Geometry: final body of the model. Coordinates: model frame, mm. Face numbers are marked on the shaded views. A direction names the side the tool comes from. Coordinates: 2 decimals unless noted, no trailing zeros. Order: outer loops, then holes, each group sorted by start corner. A loop starts at its lowest first (then second) coordinate and runs counter-clockwise, first axis right, second up. Notation, with made-up numbers: (60.5, 46) -> (94.5, 46) arc R16 cw to (94.5, 77) -> close; hole circle Ø4 at (52, 55.25). An arc over 180 degrees is marked (long way). Answer in a Markdown table with one row per item. Add a question column.
1) Ray query, line 1 (X direction, y = -0.75, z = -18); line 2 (X direction, y = -2, z = -5); line 3 (Z direction, x = 59, y = -7). Return the intervals inside material, ascending. Write a range as from..to.
2) Section query A-A on x = -10.5. Return the cut outline in (y, z) (3 decimals), then the cut area to 3 significant figures.
3) Section query B-B on x = -40.5. Return the cut outline in (y, z) (3 decimals), then the cut area to 3 significant figures.
4) Section query C-C on z = -12.5. Count the separate pieces of the cut face and the enclosed holes in it, then the cut area to 3 significant figures.
5) Contact query for flat-ended pins moving along their axis: P1, Ø8, axis at x = -64.17, y = -2.89, coming from the -Z side; P2, Ø0.7, axis at x = 122.5, z = -12, coming from the +Y side (3 decimals); P3, Ø1.5, axis at x = -33, z = -14, coming from the +Y side (3 decimals). Output: stop coordinate, or through.
6) Set-up query: the marked faces 1, 2 and 3. Return all of +Z, -Z, +X, -X, +Y, -Y with unobstructed straight access to the full face (end or side cutting, diameter ignored); none if empty.
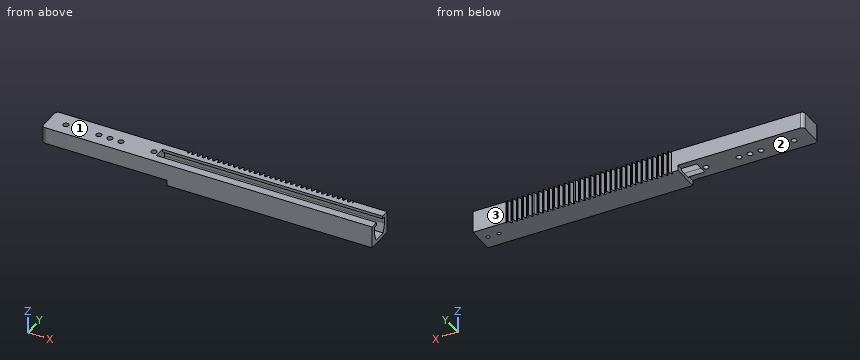
```python
from build123d import *

# Parameters (mm, degrees)
BLANKSKE_W              = 150
BLANKSKE_H              = 11.5
BLANK_DEPTH             = 20
TOOTHCUTSIM_DEPTH       = 152.763796737
TEETHCUTS_COUNT         = 33
TEETHCUTS_PITCH         = 4.712388975
BOSS_EXTRUDE1_DEPTH     = 20
BOSS_EXTRUDE2_DEPTH     = 20
SKETCH3_W               = 190
SKETCH3_H               = 20
BOSS_EXTRUDE3_DEPTH     = 14.285
CUT_EXTRUDE1_DEPTH      = 192.583040024
SKETCH6_W               = 20
SKETCH6_H               = 24.61
BOSS_EXTRUDE4_DEPTH     = 140
BOSS_EXTRUDE5_DEPTH     = 10
SKETCH9_R               = 2.5
CUT_EXTRUDE2_DEPTH      = 182.670199056
CUT_EXTRUDE5_DEPTH      = 341.88716788
CUT_EXTRUDE5_DEPTH_BACK = 154
SKETCH15_W              = 2.5
SKETCH15_H              = 15
BOSS_EXTRUDE9_DEPTH     = 10
SKETCH16_R              = 2
CUT_EXTRUDE7_DEPTH      = 10
SKETCH17_W              = 15
SKETCH17_H              = 10
CUT_EXTRUDE8_DEPTH      = 177
SKETCH20_W              = 15
SKETCH20_H              = 24.61
CUT_EXTRUDE9_DEPTH      = 40
FILLET2_R               = 3
SKETCH21_R              = 1.6
CUT_EXTRUDE10_DEPTH     = 40


with BuildPart() as part:
    # BlankSke → Blank (new body)
    with BuildSketch(Plane.XY):
        with Locations((75, 5.75)):
            Rectangle(BLANKSKE_W, BLANKSKE_H)
    extrude(amount=-BLANK_DEPTH)

    # TooCutSkeSim → ToothCutSim (cut, through all)
    with BuildSketch(Plane.XY):
        Polygon((0.654653055, 8.125), (-0.654653055, 8.125), (-1.892297439, 11.5254), (1.892297439, 11.5254), align=None)
    toothcutsim = extrude(amount=-TOOTHCUTSIM_DEPTH, mode=Mode.SUBTRACT)

    # TeethCuts: ToothCutSim ×33
    with Locations(*[(i * TEETHCUTS_PITCH, 0, 0) for i in range(1, TEETHCUTS_COUNT)]):
        add(toothcutsim, mode=Mode.SUBTRACT)

    # Sketch1 → Boss-Extrude1 (add)
    with BuildSketch(Plane(origin=(150, 0, 0), x_dir=(0, 0, -1), z_dir=(1, 0, 0))):
        Polygon((0, 8.514576213), (0, 10.714576213), (20, 10.714576213), (20, 0), (0, 0), align=None)
    extrude(amount=BOSS_EXTRUDE1_DEPTH)

    # Sketch2 → Boss-Extrude2 (add)
    with BuildSketch(Plane.ZY):
        Polygon((-20, 8.125), (-20, 10.325), (0, 10.325), (0, 0), (-20, 0), align=None)
    extrude(amount=BOSS_EXTRUDE2_DEPTH)

    # Sketch3 → Boss-Extrude3 (add)
    with BuildSketch(Plane.XZ):
        with Locations((75, -10)):
            Rectangle(SKETCH3_W, SKETCH3_H)
    extrude(amount=BOSS_EXTRUDE3_DEPTH)

    # Sketch4 → Cut-Extrude1 (cut, through all)
    with BuildSketch(Plane(origin=(170, 0, 0), x_dir=(0, 0, -1), z_dir=(1, 0, 0))):
        Polygon((2.5, -6.785211894), (2.5, -10.385211894), (8.7, -10.385211894), (16.7, -7.785211894), (16.7, -1.785211894), (16.7, 4.214788106), (8.7, 6.814788106), (2.5, 6.814788106), (2.5, 3.214788106), (0, 3.214788106), (0, -1.785211894), (0, -6.785211894), align=None)
    extrude(amount=-CUT_EXTRUDE1_DEPTH, mode=Mode.SUBTRACT)

    # Sketch6 → Boss-Extrude4 (add)
    with BuildSketch(Plane.ZY.offset(20)):
        with Locations((-10, -1.98)):
            Rectangle(SKETCH6_W, SKETCH6_H)
    extrude(amount=BOSS_EXTRUDE4_DEPTH)

    # Sketch8 → Boss-Extrude5 (add)
    with BuildSketch(Plane(origin=(170, 0, 0), x_dir=(0, 0, -1), z_dir=(1, 0, 0))):
        Polygon((20, 10.714576213), (20, -14.285), (0, -14.285), (0, -6.785211894), (2.5, -6.785211894), (2.5, -10.385211894), (8.7, -10.385211894), (16.7, -7.785211894), (16.7, 4.214788106), (8.7, 6.814788106), (2.5, 6.814788106), (2.5, 3.214788106), (0, 3.214788106), (0, 10.714576213), align=None)
    extrude(amount=BOSS_EXTRUDE5_DEPTH)

    # Sketch9 → Cut-Extrude2 (cut, through all)
    with BuildSketch(Plane(origin=(0, 0, -20), x_dir=(-1, 0, 0), z_dir=(0, 0, -1))):
        with Locations((24.169323408, -2.889762756)):
            Circle(SKETCH9_R)
        with Locations((54.169323408, -2.889762756)):
            Circle(SKETCH9_R)
        with Locations((64.169323408, -2.889762756)):
            Circle(SKETCH9_R)
        with Locations((74.169323408, -2.889762756)):
            Circle(SKETCH9_R)
        with Locations((104.169323408, -2.889762756)):
            Circle(SKETCH9_R)
    extrude(amount=-CUT_EXTRUDE2_DEPTH, mode=Mode.SUBTRACT)

    # Sketch10 → Cut-Extrude5 (cut, two sides: drawn at the far end of the back side and taken through both)
    with BuildSketch(Plane.ZY.offset(160).offset(-CUT_EXTRUDE5_DEPTH_BACK)):
        Polygon((-20, -14.285), (-15, -14.285), (-15, 10.325), (-15, 11.5), (-20, 11.5), (-20, 10.325), align=None)
    extrude(amount=CUT_EXTRUDE5_DEPTH + CUT_EXTRUDE5_DEPTH_BACK, mode=Mode.SUBTRACT)

    # Sketch15 → Boss-Extrude9 (add)
    with BuildSketch(Plane.XZ.offset(14.285)):
        with Locations((-11.17642258, -7.5)):
            Rectangle(SKETCH15_W, SKETCH15_H)
    extrude(amount=BOSS_EXTRUDE9_DEPTH)

    # Sketch16 → Cut-Extrude7 (cut)
    with BuildSketch(Plane.ZY.offset(12.42642258)):
        with Locations((-11.25, -19.285)):
            Circle(SKETCH16_R)
        with Locations((-3.75, -19.285)):
            Circle(SKETCH16_R)
    extrude(amount=-CUT_EXTRUDE7_DEPTH, mode=Mode.SUBTRACT)

    # Sketch17 → Cut-Extrude8 (cut)
    with BuildSketch(Plane.ZY.offset(160)):
        with Locations((-7.5, -19.285)):
            Rectangle(SKETCH17_W, SKETCH17_H)
    extrude(amount=-CUT_EXTRUDE8_DEPTH, mode=Mode.SUBTRACT)

    # Sketch20 → Cut-Extrude9 (cut)
    with BuildSketch(Plane.ZY.offset(160)):
        with Locations((-7.5, -1.98)):
            Rectangle(SKETCH20_W, SKETCH20_H)
    extrude(amount=-CUT_EXTRUDE9_DEPTH, mode=Mode.SUBTRACT)

    # Fillet2
    fillet2_edges = [part.edges().sort_by_distance(p)[0] for p in [
        (-120, -14.285, -7.5),
        (-120, 10.325, -7.5),
    ]]
    fillet(fillet2_edges, radius=FILLET2_R)

    # Sketch21 → Cut-Extrude10 (cut)
    with BuildSketch(Plane(origin=(0, 0, -20), x_dir=(-1, 0, 0), z_dir=(0, 0, -1))):
        with Locations((-172.560963077, -0.785239005)):
            Circle(SKETCH21_R)
        with Locations((-162.560967794, -0.785233109)):
            Circle(SKETCH21_R)
    extrude(amount=-CUT_EXTRUDE10_DEPTH, mode=Mode.SUBTRACT)


solid = part.part
```
Result:
| question | item | result |
|---|---|---|
| 1 | line 1 | -6..160.96, 164.16..170.96, 174.16..180 |
| 1 | line 2 | -120..-106.51, -101.83..-76.51, -71.83..-66.51, -61.83..-56.51, -51.83..-26.51, -21.83..-20 |
| 1 | line 3 | -20..-16.7, -2.5..0 |
| 2 | outline | (-14.285, -15) -> (-8.338, -15) -> (-10.385, -8.7) -> (-10.385, -2.5) -> (-6.785, -2.5) -> (-6.785, 0) -> (-14.285, 0) -> close; (3.215, -2.5) -> (6.815, -2.5) -> (6.815, -8.7) -> (4.767, -15) -> (10.325, -15) -> (10.325, 0) -> (3.215, 0) -> close |
| 2 | area | 142 mm2 |
| 3 | outline | (-14.285, -15) -> (10.325, -15) -> (10.325, 0) -> (-14.285, 0) -> close |
| 3 | area | 369 mm2 |
| 4 | separate pieces | 1 |
| 4 | enclosed holes | 5 |
| 4 | area | 4,250 mm2 |
| 5 | P1 | z = -15 |
| 5 | P2 | y = 8.125 |
| 5 | P3 | y = 10.325 |
| 6 | face 1 | +Z, +X, -X, +Y, -Y |
| 6 | face 2 | -Z, -X, +Y, -Y |
| 6 | face 3 | +Z, -Z, +X, +Y |
